Answer from the drawing. Dimensions are ordinates in mm from the lowest x, y and z of the part. Round coordinates to 2 decimals unless told otherwise and drop trailing zeros. Write each loop counter-clockwise with the first axis right and the second up, starting at its lowest first coordinate (ties: lowest second). Pieces come first, ordered by that corner, then holes. Notation, with made-up numbers: (3.5, 75.5) - (24.5, 75.5) arc R10 cw to (24.5, 83.5) - close; hole circle Ø11 at (67, 77.25). An arc over 180 degrees is marked (long way). Use a Markdown table: item, result. Add a question column.
1) A cutting plane is placed at B-B (z = 13). Give the vertices of the cut face in (x, y).
2) A cutting plane is placed at C-C (x = 1.4). Give the vertices of the cut face in (y, z) (3 decimals), then the cut area to 3 significant figures.
3) A cutting plane is placed at A-A (y = 23). Give the vertices of the cut face in (x, z), then the cut area to 3 significant figures.
4) This flat-tipped pin is pushed along its axis until it touches: P1, Ø6.5, axis at y = 39.245, z = 28, coming from the +X side. Where does it stop, or does it pass through?
5) Find the intervals of material crossed by probe 1 along Y at (x, z) = (1.8, 30.5); probe 2 along Z at (x, y) = (0.45, 28.5); probe 3 along Y at (x, z) = (1.3, 29.5), in increasing order. Write a range as from..to.
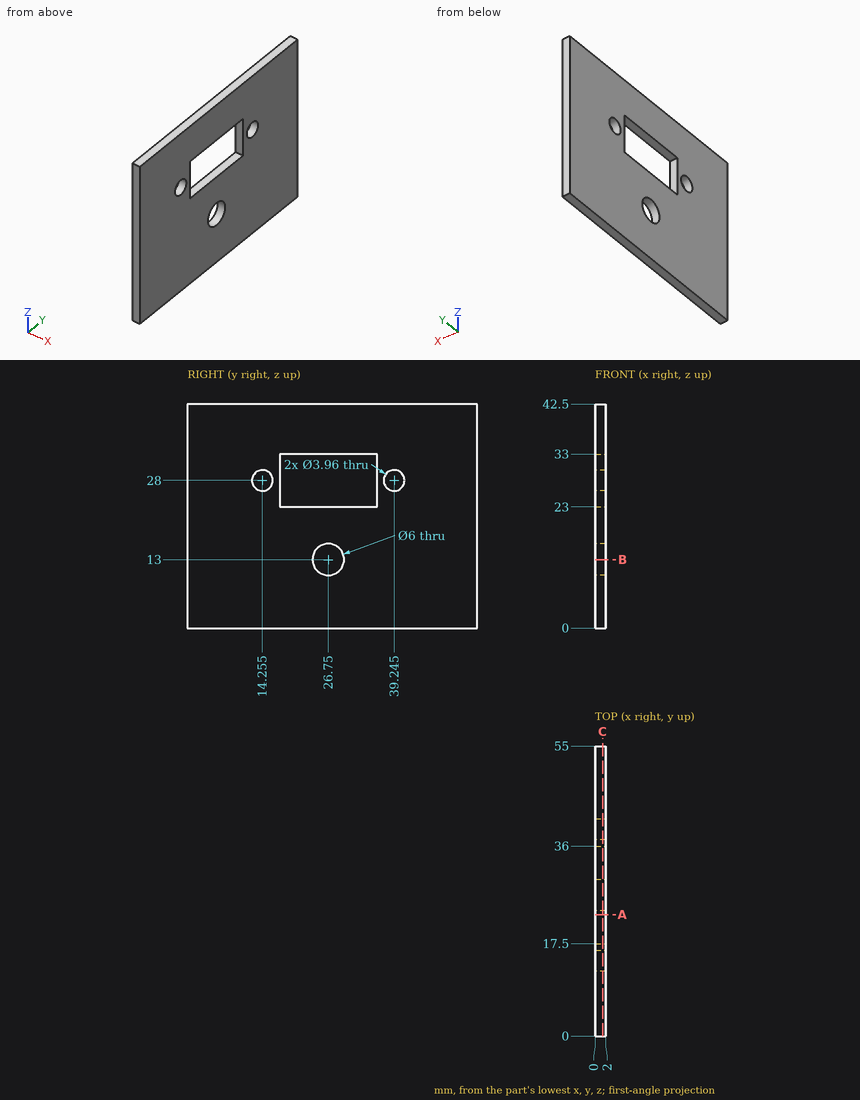
Entries:
| question | item | result |
|---|---|---|
| 1 | outline | (0, 0) - (2, 0) - (2, 23.75) - (0, 23.75) - close; (0, 29.75) - (2, 29.75) - (2, 55) - (0, 55) - close |
| 2 | outline | (0, 0) - (55, 0) - (55, 42.5) - (0, 42.5) - close; hole circle Ø3.96 at (14.255, 28); hole (17.5, 23) - (36, 23) - (36, 33) - (17.5, 33) - close; hole circle Ø6 at (26.75, 13); hole circle Ø3.96 at (39.245, 28) |
| 2 | area | 2,100 mm² |
| 3 | outline | (0, 0) - (2, 0) - (2, 23) - (0, 23) - close; (0, 33) - (2, 33) - (2, 42.5) - (0, 42.5) - close |
| 3 | area | 65.0 mm² |
| 4 | P1 | stops at x = 2 |
| 5 | probe 1 | y = 0..17.5, 36..55 |
| 5 | probe 2 | z = 0..10.56, 15.44..23, 33..42.5 |
| 5 | probe 3 | y = 0..12.96, 15.55..17.5, 36..37.95, 40.54..55 |
